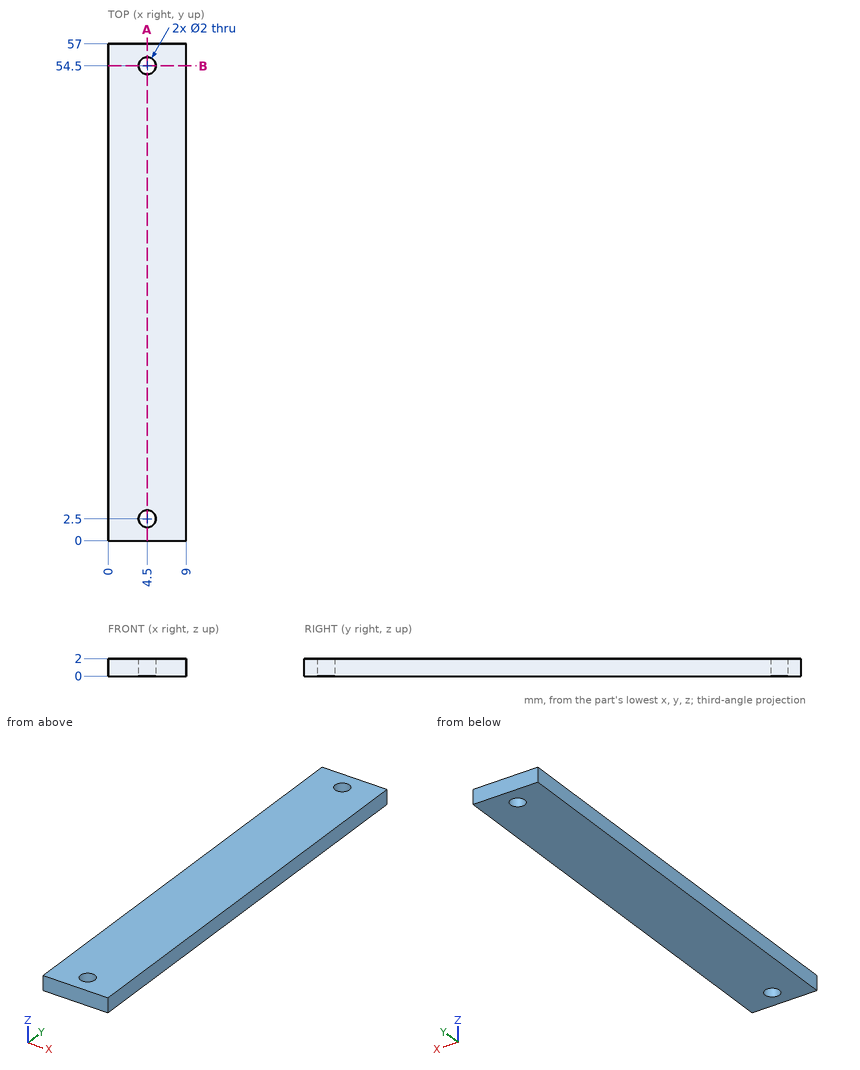
Geometry: see drawing. Coordinates: mm, zero at the bounding-box minimum. Round coordinates to 2 decimals unless told otherwise and drop trailing zeros. Write each loop counter-clockwise with the first axis right and the second up, starting at its lowest first coordinate (ties: lowest second). Pieces come first, ordered by that corner, then holes. Notation, with made-up numbers: (10.5, 86.5) - (26.5, 86.5) arc R17 cw to (26.5, 112.5) - close; hole circle Ø2 at (33, 3). An arc over 180 degrees is marked (long way). Use CSV: the item, a comma, the result in double quotes. Start each with the question number.
(1) First-contact query: pin 1 Ø1.6 at (x, y) = (4.5, 54.5) entering from -Z. Flat tip, straight axial feed; report the tip coordinate or a pass-through.
(2) Cut plane A-A, the plane x = 4.5. Return loops of the section in (y, z).
(3) Material intervals for probe 1 along Y at (x, z) = (4.5, 1.05); probe 2 along X at (y, z) = (2.5, 0.6), sorted ascending. Write a range as [from, to].
(4) Cut plane B-B, the plane y = 54.5. Return loops of the section in (x, z), and give its area (3 significant figures).
Geometry says:
1,pin 1,"through"
2,outline,"(0, 0) - (1.5, 0) - (1.5, 2) - (0, 2) - close; (3.5, 0) - (53.5, 0) - (53.5, 2) - (3.5, 2) - close; (55.5, 0) - (57, 0) - (57, 2) - (55.5, 2) - close"
3,probe 1,"[0, 1.5], [3.5, 53.5], [55.5, 57]"
3,probe 2,"[0, 3.5], [5.5, 9]"
4,outline,"(0, 0) - (3.5, 0) - (3.5, 2) - (0, 2) - close; (5.5, 0) - (9, 0) - (9, 2) - (5.5, 2) - close"
4,area,"14.0 mm²"
